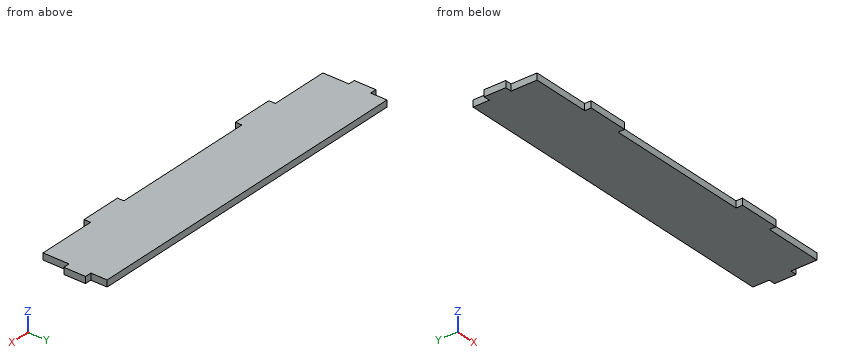
```python
from build123d import *

# Parameters (mm, degrees)
ESQUISSE1_W             = 330
ESQUISSE1_H             = 65
BOSS_EXTRU_1_DEPTH      = 6
ESQUISSE2_W             = 134
ESQUISSE2_H             = 6
ESQUISSE2_W_2           = 6
ESQUISSE2_H_2           = 15
ENL_V_MAT_EXTRU_1_DEPTH = 6


with BuildPart() as part:
    # Esquisse1 → Boss.-Extru.1 (new body)
    with BuildSketch(Plane.XY):
        with Locations((-165, 32.5)):
            Rectangle(ESQUISSE1_W, ESQUISSE1_H)
    extrude(amount=BOSS_EXTRU_1_DEPTH)

    # Esquisse2 → Enlèv. mat.-Extru.1 (cut)
    with BuildSketch(Plane.XY.offset(6)):
        Polygon((-330, 0), (-270, 0), (-270, 6), (-324, 6), (-324, 30), (-330, 30), align=None)
        Polygon((0, 0), (-60, 0), (-60, 6), (-6, 6), (-6, 30), (0, 30), align=None)
        with Locations((-165, 3)):
            Rectangle(ESQUISSE2_W, ESQUISSE2_H)
        with Locations((-327, 57.5)):
            Rectangle(ESQUISSE2_W_2, ESQUISSE2_H_2)
        with Locations((-3, 57.5)):
            Rectangle(ESQUISSE2_W_2, ESQUISSE2_H_2)
    extrude(amount=-ENL_V_MAT_EXTRU_1_DEPTH, mode=Mode.SUBTRACT)


solid = part.part
```
Work out the finished part from the listing and answer in its coordinate system (mm). Give positions to 0.01 mm unless a question says otherwise; leave off trailing zeros. Write each loop counter-clockwise with the first axis right and the second up, starting at its lowest first coordinate (ties: lowest second). Pieces come first, ordered by that corner, then holes. Notation, with made-up numbers: (18, 10.25) -> (43, 10.25) arc R23 cw to (43, 40.25) -> close; hole circle Ø1 at (39.5, 48). An arc over 180 degrees is marked (long way). Write item = value, one per line.
Q1. Section C-C on x = -210.5 is taken. Determine the outline of the cut face in (y, z).
Computed values:
outline = (6, 0) -> (65, 0) -> (65, 6) -> (6, 6) -> close
Q2. Section A-A on z = 0.95 is taken. Determine the outline of the cut face in (x, y).
Computed values:
outline = (-330, 30) -> (-324, 30) -> (-324, 6) -> (-270, 6) -> (-270, 0) -> (-232, 0) -> (-232, 6) -> (-98, 6) -> (-98, 0) -> (-60, 0) -> (-60, 6) -> (-6, 6) -> (-6, 30) -> (0, 30) -> (0, 50) -> (-6, 50) -> (-6, 65) -> (-324, 65) -> (-324, 50) -> (-330, 50) -> close
Q3. Consider line 1 along X through (y, z) = (53, 1.15); line 2 along Y through (x, z) = (-230, 3.95); line 3 along X through (y, z) = (4.5, 2.8). Determine where each line is inside the solid, lowest interval first.
Computed values:
line_1 = -324 to -6
line_2 = 6 to 65
line_3 = -270 to -232, -98 to -60
Q4. Section B-B on y = 15 is taken. Determine the outline of the cut face in (x, z), and give its area (3 significant figures).
Computed values:
outline = (-324, 0) -> (-6, 0) -> (-6, 6) -> (-324, 6) -> close
area = 1,910 mm^2
Q5. Flat-ended cylindrical pins translate along their axes: pin 1 Ø1.8 at (y, z) = (3.5, 3.5) entering from +X; pin 2 Ø3 at (x, z) = (-326.5, 3.5) entering from +Y; pin 3 Ø3 at (x, z) = (-29, 2) entering from -Y. Find the tip coordinate at first contact, or state that the pin passes through.
Computed values:
pin_1 = -60
pin_2 = 50
pin_3 = 6
